Source: CAD feature listing. Evaluate the final solid. Frame: model axes, mm. A direction names the side the tool comes from. Round coordinates to 2 decimals unless told otherwise and drop trailing zeros. Write each loop counter-clockwise with the first axis right and the second up, starting at its lowest first coordinate (ties: lowest second). Pieces come first, ordered by that corner, then holes. Notation, with made-up numbers: M -10,-10.5 L 21,-10.5 A7 ccw 21,-4.5 Z; hole C -17.5,35.5 d9. An arc over 180 degrees is marked long. Answer in a Markdown table with one row per item.
from build123d import *

# Parameters (mm, degrees)
F0_W     = 80
F0_H     = 50
F1_DEPTH = 10
F3_DEPTH = 15
F4_R     = 5


with BuildPart() as f1:
    # F0 (on Top) → F1 (new body)
    with BuildSketch(Plane.XY):
        Rectangle(F0_W, F0_H)
    extrude(amount=F1_DEPTH)

    # F2 (on face) → F3 (cut)
    with BuildSketch(Plane.XY.offset(10)):
        Polygon((25, -5.773503), (30, -2.886751), (30, 2.886751), (25, 5.773503), (20, 2.886751), (20, -2.886751), align=None)
    extrude(amount=-F3_DEPTH, mode=Mode.SUBTRACT)

    # F4
    f4_edges = [f1.edges().sort_by_distance(p)[0] for p in [
        (0, -25, 10),
        (40, 0, 10),
        (0, 25, 10),
        (-40, 0, 10),
    ]]
    fillet(f4_edges, radius=F4_R)


solid = f1.part
Q1. Section D-D (x = -3). Return loops of the section in (y, z), and give its area (3 significant figures).
Solutions:
| item | result |
|---|---|
| outline | M -25,0 L 25,0 L 25,5 A5 ccw 20,10 L -20,10 A5 ccw -25,5 Z |
| area | 489 mm2 |
Q2. Material intervals for probe 1 along X at (y, z) = (-1.5, 3); probe 2 along Y at (x, z) = (25, 6); probe 3 along X at (y, z) = (5, 3.5), sorted ascending.
Solutions:
| item | result |
|---|---|
| probe 1 | x = -40 to 20, 30 to 40 |
| probe 2 | y = -24.9 to -5.77, 5.77 to 24.9 |
| probe 3 | x = -40 to 23.66, 26.34 to 40 |
Q3. Access query for faces 1 (the cylindrical face through (-39, 0, 8)), 2 (the flat face through (30, 0, 5)). Directions: +Z, -Z, +X, -X, +Y, -Y. A direction counts if a zero-diameter tool reaches every point of the face in a straight line with its end or side. Return the directions, or none.
Solutions:
| item | result |
|---|---|
| face 1 | +Z, -X, +Y, -Y |
| face 2 | +Z, -Z |
Q4. Contact query for a flat-ended pin moving along its axis: pin 1 Ø10 at (x, y) = (-6.5, 10) entering from -Z. Output: stop coordinate, or through.
Solutions:
| item | result |
|---|---|
| pin 1 | stops at z = 0 |
Q5. Section C-C (x = 28.5). Return loops of the section in (y, z), and give its area (3 significant figures).
Solutions:
| item | result |
|---|---|
| outline | M -25,0 L -3.75,0 L -3.75,10 L -20,10 A5 ccw -25,5 Z; M 3.75,0 L 25,0 L 25,5 A5 ccw 20,10 L 3.75,10 Z |
| area | 414 mm2 |
Q6. Section A-A (z = 3). Return loops of the section in (x, y).
Solutions:
| item | result |
|---|---|
| outline | M -40,-25 L 40,-25 L 40,25 L -40,25 Z; hole M 20,-2.89 L 25,-5.77 L 30,-2.89 L 30,2.89 L 25,5.77 L 20,2.89 Z |
Q7. Pull-direction query (X, two-part tool) for faces 3 (the cylindrical face through (38, 0, 9)), 4 (the flat face through (-1, 0, 0)), 5 (the flat face through (20, 0, 5)); classes: pulls with the +X half, pulls with the -X half, needs draft (parallel to the pull), parting line crosses it, or undercut.
Solutions:
| item | result |
|---|---|
| face 3 | pulls with the +X half |
| face 4 | needs draft |
| face 5 | undercut |
Q8. Section B-B (y = -0.5). Return loops of the section in (x, z).
Solutions:
| item | result |
|---|---|
| outline | M -40,0 L 20,0 L 20,10 L -35,10 A5 ccw -40,5 Z; M 30,0 L 40,0 L 40,5 A5 ccw 35,10 L 30,10 Z |
